Build history of the part. All positions in model axes, mm. Face numbers are marked on the shaded views. Give positions to 0.01 mm unless a question says otherwise; leave off trailing zeros. Write each loop counter-clockwise with the first axis right and the second up, starting at its lowest first coordinate (ties: lowest second). Pieces come first, ordered by that corner, then holes. Notation, with made-up numbers: (-26, 47) -> (-7, 47) arc R15 ccw to (-7, 60) -> close; hole circle Ø7 at (19, -15.5). An arc over 180 degrees is marked (long way). Write item = value, one per line. Start each with the question number.
Q1. Drop flat-ended pins along their axis: P1, Ø1.5, axis at x = -6, y = 11, coming from the +Z side; P2, Ø6, axis at x = 0, y = 17.46, coming from the +Z side; P3, Ø2, axis at x = 5, y = 10.5, coming from the +Z side; P4, Ø15, axis at x = 11.5, z = 11, coming from the +Y side (3 decimals). Give the stop position or say it passes through.
Q2. Saw through at D-D, the plane z = -10. List the corners of the cut face in (x, y) (1 decimal).
Q3. Saw through at A-A, the plane x = 0. List the corners of the cut face in (y, z) (1 decimal), then the cut area to 3 significant figures.
Q4. Saw through at C-C, the plane y = 20.75. List the corners of the cut face in (x, z) (1 decimal), then the cut area to 3 significant figures.
Q5. Wall check: line 1 (Y direction, x = 0, z = 6.5) (3 decimals); line 2 (X direction, y = 5.75, z = 0); line 3 (X direction, y = 16.25, z = 0). Give the ranges that are in metal, low to high.
Q6. Saw through at B-B, the plane z = 0. List the corners of the cut face in (x, y) (1 decimal), then the cut area to 3 significant figures.
Q7. Mould opens along Z. For the marked faces 1, 2 and 3 say: pulls with the +Z half, pulls with the -Z half, needs draft (parallel to the pull), parting line crosses it, or undercut.
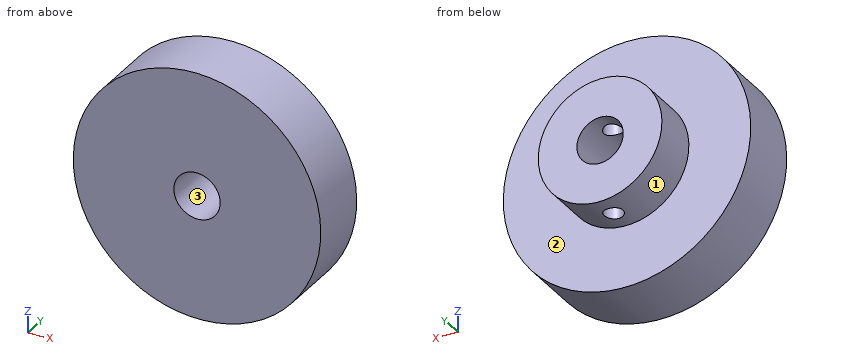
Autodesk Inventor part; units mm, degrees
ref_plane "YZ Plane" through (0, 0, 0) normal (1, 0, 0) x (0, 1, 0)
ref_plane "XZ Plane" through (0, 0, 0) normal (0, 1, 0) x (-1, 0, 0)
ref_plane "XY Plane" through (0, 0, 0) normal (0, 0, 1) x (1, 0, 0)
sketch "Sketch1" plane through (0, 0, 0) normal (1, 0, 0) x (0, 1, 0)
  line L0 (22.225, 4.7625) -> (22.225, 12.7)
  line L1 (22.225, 12.7) -> (12.7, 12.7)
  line L2 (12.7, 12.7) -> (12.7, 25.4)
  line L3 (12.7, 25.4) -> (0, 25.4)
  line L4 (0, 25.4) -> (0, 4.7625)
  line L5 (0, 4.7625) -> (22.225, 4.7625)
  line L6 (-4.445, 0) -> (26.67, 0)
  line L7 (0, -5.08) -> (0, 30.48) construction
  point P0 (0, 0)
  dimension "d0" = 25.4
  dimension "d1" = 9.525
  dimension "d2" = 22.225
  dimension "d4" = 12.7
  dimension "d5" = 50.8
revolve "Revolution1" add sketch "Sketch1" angle 360 about axis through (0, -10, 0) along (0, 1, 0)
sketch "Sketch2" plane through (0, 22.225, 0) normal (0, 1, 0) x (1, 0, 0)
  circle A0 centre (0, 0) radius 12.7
  point P0 (0, -12.7)
ref_plane "Work Plane1" through (0, 22.225, 12.7) normal (0, 0, 1) x (1, 0, 0)
sketch "Sketch3" plane through (0, 22.225, 12.7) normal (0, 0, 1) x (1, 0, 0)
  line L0 (12.7, 0) -> (-12.7, 0)
  point P0 (0, -22.225)
  point P1 (0, -4.7625)
  dimension "d7" = 4.7625
hole "Hole1" at (0, 17.4625, 12.7) direction (0, 0, -1) diameter 3.8608 end through all
properties part number "Clamp Knob" material "Iron, Cast"
Report:
q1.P1 = 24.85
q1.P2 = 12.7
q1.P3 = 25.08
q1.P4 = 22.225
q2.outline = (-23.3, 0) -> (23.3, 0) -> (23.3, 12.7) -> (7.8, 12.7) -> (7.8, 22.2) -> (-7.8, 22.2) -> (-7.8, 12.7) -> (-23.3, 12.7) -> close; hole circle Ø3.9 at (0, 17.5)
q3.outline = (0, -25.4) -> (12.7, -25.4) -> (12.7, -12.7) -> (15.5, -12.7) -> (15.5, -4.8) -> (0, -4.8) -> close; (0, 4.8) -> (15.5, 4.8) -> (15.5, 12.7) -> (12.7, 12.7) -> (12.7, 25.4) -> (0, 25.4) -> close; (19.4, -12.7) -> (22.2, -12.7) -> (22.2, -4.8) -> (19.4, -4.8) -> close; (19.4, 4.8) -> (22.2, 4.8) -> (22.2, 12.7) -> (19.4, 12.7) -> close
q3.area = 614 mm2
q4.outline = circle Ø25.4 at (0, 0); hole circle Ø9.5 at (0, 0)
q4.area = 435 mm2
q5.line_1 = 0 to 15.532, 19.393 to 22.225
q5.line_2 = -25.4 to -4.76, 4.76 to 25.4
q5.line_3 = -12.7 to -4.76, 4.76 to 12.7
q6.outline = (-25.4, 0) -> (-4.8, 0) -> (-4.8, 22.2) -> (-12.7, 22.2) -> (-12.7, 12.7) -> (-25.4, 12.7) -> close; (4.8, 0) -> (25.4, 0) -> (25.4, 12.7) -> (12.7, 12.7) -> (12.7, 22.2) -> (4.8, 22.2) -> close
q6.area = 675 mm2
q7.face_1 = parting line crosses it
q7.face_2 = needs draft
q7.face_3 = undercut
